Work out the finished part from the listing and answer in its coordinate system (mm). A direction names the side the tool comes from. Coordinates: 2 decimals unless noted, no trailing zeros. Write each loop counter-clockwise with the first axis right and the second up, starting at its lowest first coordinate (ties: lowest second). Pieces come first, ordered by that corner, then holes. Notation, with made-up numbers: (-35, -21) - (5, -21) arc R12 cw to (5, -4) - close; hole circle Ø3 at (67.25, 51.25). An arc over 180 degrees is marked (long way). One line per item, written item: value.
```python
from build123d import *

# Parameters (mm, degrees)
F0_W     = 99
F0_H     = 99
F1_DEPTH = 3
F2_R     = 26
F2_R_2   = 23
F3_DEPTH = 4
F4_R     = 26
F4_R_2   = 24.5
F5_DEPTH = 60
F6_W     = 99
F6_H     = 99
F6_W_2   = 96
F6_H_2   = 96
F7_DEPTH = 30
F8_R     = 2.5
F9_DEPTH = 25


with BuildPart() as f1:
    # F0 (on Front) → F1 (new body)
    with BuildSketch(Plane.XZ):
        Rectangle(F0_W, F0_H)
    extrude(amount=-F1_DEPTH)

    # F2 (on Front) → F3 (cut)
    with BuildSketch(Plane.XZ):
        Circle(F2_R)
        Circle(F2_R_2, mode=Mode.SUBTRACT)
        Circle(F2_R_2)
    extrude(amount=-F3_DEPTH, mode=Mode.SUBTRACT)

    # F4 (on face) → F5 (join)
    with BuildSketch(Plane.XZ):
        Circle(F4_R)
        Circle(F4_R_2, mode=Mode.SUBTRACT)
    extrude(amount=-F5_DEPTH)

    # F6 (on Front) → F7 (join)
    with BuildSketch(Plane.XZ):
        Rectangle(F6_W, F6_H)
        Rectangle(F6_W_2, F6_H_2, mode=Mode.SUBTRACT)
    extrude(amount=F7_DEPTH)

    # F8 (on face) → F9 (cut)
    with BuildSketch(Plane.YZ.offset(-48)):
        with Locations((-15, -24.5450405731)):
            Circle(F8_R)
    extrude(amount=-F9_DEPTH, mode=Mode.SUBTRACT)


solid = f1.part
```
Item 1: Which of the six approach directions +Z, -Z, +X, -X, +Y, -Y give full straight-line access (tool end or side, diameter ignored) to faces 4 (the face through (-48, -15, -1)), 5 (the face through (13.17, 29.58, 20.66)), 6 (the face through (-48.74, -16.98, -26.07))?
Evaluation:
face 4: -Y
face 5: +Y, -Y
face 6: -X
Item 2: Given pin 1 (12 mm diameter, centred on x = 4.5, z = 12.5, fed in from -Y); pin 2 (6 mm diameter, centred on y = 6.5, z = 7.5, fed in from -X); pin 3 (3 mm diameter, centred on x = -8.5, z = -37.5, fed in from -Y); pin 4 (10 mm diameter, centred on y = 48.5, z = 6, fed in from +X), each flat-ended and moving along its own axis, determine where each tip first touches the part or whether it passes through.
Evaluation:
pin 1: passes through
pin 2: stops at x = -25.61
pin 3: stops at y = 0
pin 4: stops at x = 25.98
Item 3: Determine the mould class of faces 1 (the face through (21, 3, 23)), 2 (the face through (48, -15, -1)), 3 (the face through (-20.633, 31.101, -15.821)) for opening direction X: +X half, -X half, draft (parallel to the pull), parting line (faces both ways), or undercut.
Evaluation:
face 1: draft
face 2: undercut
face 3: parting line
Item 4: Section A-A, the plane x = 0 is taken. Determine the outline of the cut face in (y, z), then the cut area to 3 significant figures.
Evaluation:
outline: (-30, -49.5) - (3, -49.5) - (3, -26) - (60, -26) - (60, -24.5) - (0, -24.5) - (0, -48) - (-30, -48) - close; (-30, 48) - (0, 48) - (0, 24.5) - (60, 24.5) - (60, 26) - (3, 26) - (3, 49.5) - (-30, 49.5) - close
area: 411 mm2
Item 5: Section B-B, the plane z = 0 is taken. Determine the outline of the cut face in (x, y).
Evaluation:
outline: (-49.5, -30) - (-48, -30) - (-48, 0) - (-24.5, 0) - (-24.5, 60) - (-26, 60) - (-26, 3) - (-49.5, 3) - close; (24.5, 0) - (48, 0) - (48, -30) - (49.5, -30) - (49.5, 3) - (26, 3) - (26, 60) - (24.5, 60) - close
Item 6: Section C-C, the plane y = -19 is taken. Determine the outline of the cut face in (x, z), then the cut area to 3 significant figures.
Evaluation:
outline: (-49.5, -49.5) - (49.5, -49.5) - (49.5, 49.5) - (-49.5, 49.5) - close; hole (-48, -48) - (48, -48) - (48, 48) - (-48, 48) - close
area: 585 mm2
Item 7: Section D-D, the plane x = -28 is taken. Determine the outline of the cut face in (y, z).
Evaluation:
outline: (-30, -49.5) - (3, -49.5) - (3, 49.5) - (-30, 49.5) - (-30, 48) - (0, 48) - (0, -48) - (-30, -48) - close
Item 8: Consider probe 1 along Z at (x, y) = (33, -23.5); probe 2 along Z at (x, y) = (-48.3, -15). Determine where each line is inside the solid, lowest interval first.
Evaluation:
probe 1: z = -49.5 to -48, 48 to 49.5
probe 2: z = -49.5 to -27.05, -22.05 to 49.5
